from build123d import *

# Parameters (mm, degrees)
SKETCH1_W           = 50
SKETCH1_H           = 20
BOSS_EXTRUDE1_DEPTH = 10
SKETCH3_W           = 5
SKETCH3_H           = 20
BOSS_EXTRUDE2_DEPTH = 26
SKETCH4_W           = 15
SKETCH4_H           = 36
BOSS_EXTRUDE3_DEPTH = 20
BOSS_EXTRUDE4_DEPTH = 7
BOSS_EXTRUDE5_START = -7
SKETCH6_R           = 50
SKETCH6_R_2         = 4
BOSS_EXTRUDE5_DEPTH = 7
BOSS_EXTRUDE6_START = 64
BOSS_EXTRUDE6_DEPTH = 64
BOSS_EXTRUDE7_DEPTH = 5
FILLET1_R           = 5
SKETCH9_W           = 59
SKETCH9_H           = 30
BOSS_EXTRUDE8_DEPTH = 5


with BuildPart() as part:
    # Sketch1 → Boss-Extrude1 (new body)
    with BuildSketch(Plane(origin=(0, 0, 0), x_dir=(1, 0, 0), z_dir=(0, 1, 0))):
        with Locations((25, 10)):
            Rectangle(SKETCH1_W, SKETCH1_H)
    extrude(amount=BOSS_EXTRUDE1_DEPTH)

    # Sketch3 → Boss-Extrude2 (add)
    with BuildSketch(Plane(origin=(0, 10, 0), x_dir=(1, 0, 0), z_dir=(0, 1, 0))):
        with Locations((2.5, 10)):
            Rectangle(SKETCH3_W, SKETCH3_H)
        with Locations((47.5, 10)):
            Rectangle(SKETCH3_W, SKETCH3_H)
    extrude(amount=BOSS_EXTRUDE2_DEPTH)

    # Sketch4 → Boss-Extrude3 (add)
    with BuildSketch(Plane(origin=(0, 0, -20), x_dir=(-1, 0, 0), z_dir=(0, 0, -1))):
        with Locations((-52.5, 18)):
            Rectangle(SKETCH4_W, SKETCH4_H)
    extrude(amount=-BOSS_EXTRUDE3_DEPTH)

    # Sketch5 → Boss-Extrude4 (add)
    with BuildSketch(Plane(origin=(60, 0, 0), x_dir=(0, 0, -1), z_dir=(1, 0, 0))):
        with BuildLine():
            Line((10, 37.5), (10, 36))
            Line((10, 36), (20, 36))
            Line((20, 36), (20, 47.5))
            ThreePointArc((20, 47.5), (17.071067812, 40.428932188), (10, 37.5))
        make_face()
        with BuildLine():
            ThreePointArc((0, 47.5), (2.928932188, 40.428932188), (10, 37.5))
            Line((10, 37.5), (10, 43.5))
            ThreePointArc((10, 43.5), (7.171572875, 44.671572875), (6, 47.5))
            Line((6, 47.5), (0, 47.5))
        make_face()
        with BuildLine():
            Line((10, 43.5), (10, 37.5))
            ThreePointArc((10, 37.5), (17.071067812, 40.428932188), (20, 47.5))
            Line((20, 47.5), (14, 47.5))
            ThreePointArc((14, 47.5), (12.828427125, 44.671572875), (10, 43.5))
        make_face()
        with BuildLine():
            Line((0, 36), (10, 36))
            Line((10, 36), (10, 37.5))
            ThreePointArc((10, 37.5), (2.928932188, 40.428932188), (0, 47.5))
            Line((0, 47.5), (0, 36))
        make_face()
        with BuildLine():
            ThreePointArc((20, 47.5), (10, 57.5), (0, 47.5))
            Line((0, 47.5), (6, 47.5))
            ThreePointArc((6, 47.5), (10, 51.5), (14, 47.5))
            Line((14, 47.5), (20, 47.5))
        make_face()
    extrude(amount=-BOSS_EXTRUDE4_DEPTH)

    # Sketch6 → Boss-Extrude5 (add)
    with BuildSketch(Plane(origin=(60, 0, 0), x_dir=(0, 0, -1), z_dir=(1, 0, 0)).offset(BOSS_EXTRUDE5_START)):
        with Locations((10, 47.5)):
            Circle(SKETCH6_R)
        with Locations((10, 47.5)):
            Circle(SKETCH6_R_2, mode=Mode.SUBTRACT)
    extrude(amount=BOSS_EXTRUDE5_DEPTH)

    # Sketch7 → Boss-Extrude6 (add)
    with BuildSketch(Plane.ZY.offset(-53).offset(BOSS_EXTRUDE6_START)):
        with BuildLine():
            Line((-60, 47.5), (-55, 47.5))
            ThreePointArc((-55, 47.5), (-10, 2.5), (35, 47.5))
            Line((35, 47.5), (40, 47.5))
            ThreePointArc((40, 47.5), (-10, -2.5), (-60, 47.5))
        make_face()
    extrude(amount=-BOSS_EXTRUDE6_DEPTH)

    # Sketch8 → Boss-Extrude7 (add)
    with BuildSketch(Plane.ZY.offset(11)):
        with BuildLine():
            Line((-55, 47.5), (35, 47.5))
            ThreePointArc((35, 47.5), (-10, 2.5), (-55, 47.5))
        make_face()
    extrude(amount=-BOSS_EXTRUDE7_DEPTH)

    # Fillet1
    fillet1_edges = [part.edges().sort_by_distance(p)[0] for p in [
        (-11, -2.5, -10),
    ]]
    fillet(fillet1_edges, radius=FILLET1_R)

    # Sketch9 → Boss-Extrude8 (add)
    with BuildSketch(Plane(origin=(0, 47.5, 0), x_dir=(1, 0, 0), z_dir=(0, 1, 0))):
        with Locations((23.5, 40)):
            Rectangle(SKETCH9_W, SKETCH9_H)
        with Locations((23.5, -20)):
            Rectangle(SKETCH9_W, SKETCH9_H)
    extrude(amount=-BOSS_EXTRUDE8_DEPTH)


solid = part.part
Read the model definition and answer for the solid it produces. Units are mm, in the model's axes. A direction names the side the tool comes from. Coordinates: 2 decimals unless noted, no trailing zeros. Loops run counter-clockwise (first coordinate to the right, second up) from the corner with the lowest first, then second, coordinate; pieces in that order, holes last. Notation, with made-up numbers: (56.25, 42.25) - (75.25, 42.25) arc R20 cw to (75.25, 79.25) - close; hole circle Ø8 at (-15.5, -30.75). An arc over 180 degrees is marked (long way). Answer in a Markdown table with one row per item.
Q1. Straight lines are drawn through the part: line 1 along X through (y, z) = (13.5, 1); line 2 along Z through (x, y) = (1, 24); line 3 along Z through (x, y) = (3, 27.5). For each, find the intervals that lie inside material, in ascending order. Write a range as [from, to].
Here are the results:
| item | result |
|---|---|
| line 1 | x = [-11, -6], [53, 60] |
| line 2 | z = [-54.13, -48.38], [-20, 0], [28.38, 34.13] |
| line 3 | z = [-55.83, -50.31], [-20, 0], [30.31, 35.83] |
Q2. Find section B-B on y = 19. Count the separate pieces of the cut face and the enclosed holes in it, plus the area to 3 significant figures.
Here are the results:
| item | result |
|---|---|
| separate pieces | 2 |
| enclosed holes | 1 |
| area | 1,970 mm^2 |
Q3. Given P1, Ø4, axis at x = 3.5, z = -6, coming from the +Y side; P2, Ø6.5, axis at x = 50, z = -7.5, coming from the +Y side; P3, Ø2, axis at x = 26.5, y = 26.5, coming from the +Z side, each flat-ended and moving along its own axis, determine where each tip first touches the part or whether it passes through.
Here are the results:
| item | result |
|---|---|
| P1 | stops at y = 36 |
| P2 | stops at y = 97.48 |
| P3 | stops at z = 35.83 |
Q4. Find section C-C on y = 71.5. Write down the section's boundary in (x, z).
Here are the results:
| item | result |
|---|---|
| outline | (53, -53.86) - (60, -53.86) - (60, 33.86) - (53, 33.86) - close |
Q5. The mould has two halves that part along Y. Classify faces 4 (the flat face through (2, 36, -10)), 5 (the flat face through (0, 19, -10)), 6 (the flat face through (-6, 25, -9)), 7 (the flat face through (53, 62, -9)): pulls with the +Y half, pulls with the -Y half, needs draft (parallel to the pull), parting line crosses it, or undercut.
Here are the results:
| item | result |
|---|---|
| face 4 | pulls with the +Y half |
| face 5 | needs draft |
| face 6 | undercut |
| face 7 | undercut |
Q6. For faces 1 (the flat face through (5, 23, -10)), 2 (the flat face through (21, 47.5, -33)), 3 (the flat face through (23, 42.5, -40)), determine the directions among +Z, -Z, +X, -X, +Y, -Y from which every point of the face is accessible in a straight line to the end or side of a thin tool.
Here are the results:
| item | result |
|---|---|
| face 1 | +Y |
| face 2 | +Z, -Z, -X, +Y |
| face 3 | none |
Q7. Find section A-A on x = 50.5. Write down the section's boundary in (y, z), plus the area to 3 significant figures.
Here are the results:
| item | result |
|---|---|
| outline | (3.63, -20) - (36, -20) - (36, 0) - (3.63, 0) arc R45 cw to (42.5, 34.72) - (42.5, 5) - (47.5, 5) - (47.5, 40) arc R50 ccw to (47.5, -60) - (47.5, -25) - (42.5, -25) - (42.5, -54.72) arc R45 cw to start |
| area | 1,710 mm^2 |
